Check sheet for the modelled part. Datum: model origin and axes. Units: mm. A direction names the side the tool comes from. Round coordinates to 2 decimals unless told otherwise and drop trailing zeros. Write each loop counter-clockwise with the first axis right and the second up, starting at its lowest first coordinate (ties: lowest second). Pieces come first, ordered by that corner, then holes.
Item 1: Material ranges on line 1 (Y direction, x = -26, z = 45); line 2 (Z direction, x = -27.25, y = -33.5); line 3 (X direction, y = -36.5, z = 44.9), recorded low to high.
Item 2: Cross-section at A-A on x = -26. Enter the section's corners in (y, z).
Item 3: Tool access check on faces 5 (the flat face through (-23.36, -34.51, 46.49)), 6 (the cylindrical face through (-25.26, -37.42, 44.38)). Record the directions out of +Z, -Z, +X, -X, +Y, -Y that give a thin tool (end or side, any length) a straight path to the whole face; none if there is none.
Item 4: Cross-section at B-B on z = 44.3. Enter the section's corners in (x, y).
Item 5: Go/stop test with flat-tipped pins: pin 1 Ø1.5 at (y, z) = (-38.5, 46.5) entering from +X; pin 2 Ø1.5 at (x, z) = (-27.5, 45) entering from +Y; pin 3 Ø0.5 at (x, z) = (-26.5, 46.5) entering from -Y; pin 4 Ø3 at (x, y) = (-26, -36) entering from +Z. Record where each tip stops, or that it passes through.
Item 6: Release check for a two-part mould opening along Y. For faces 1 (the flat face through (-23.39, -37.54, 46.49)), 2 (the flat face through (-29, -34, 47)), 3 (the cylindrical face through (-26.521, -32.034, 44.873)), 4 (the flat face through (-28.61, -34.46, 46.49)) record: +Y half, -Y half, draft (parallel to the pull), parting line (faces both ways), or undercut.
from build123d import *

# Parameters (mm, degrees)
SKETCH182_R     = 4
SKETCH182_R_2   = 1.6
PAD075_DEPTH    = 3.2
SKETCH183_R     = 4
PAD076_DEPTH    = 1
CHAMFER032_SIZE = 0.2


with BuildPart() as part:
    # Sketch182 → Pad075 (new body)
    with BuildSketch(Plane.XY):
        Circle(SKETCH182_R)
        Circle(SKETCH182_R_2, mode=Mode.SUBTRACT)
    extrude(amount=PAD075_DEPTH)

    # Sketch183 (on Face4 of Pad075) → Pad076 (join)
    with BuildSketch(Plane.XY.offset(3.2)):
        Circle(SKETCH183_R)
        Polygon((3.5, 0), (1.75, 3.031089), (-1.75, 3.031089), (-3.5, 0), (-1.75, -3.031089), (1.75, -3.031089), align=None, mode=Mode.SUBTRACT)
    extrude(amount=PAD076_DEPTH)

    # Chamfer032
    chamfer032_edges = [part.edges().sort_by_distance(p)[0] for p in [
        (-1.6, 0, 3.2),
        (-1.6, 0, 0),
        (-4, 0, 0),
        (-4, 0, 4.2),
    ]]
    chamfer(chamfer032_edges, length=CHAMFER032_SIZE)


with BuildPart() as part_1:
    # Body049 placement: moved
    add(part.part.moved(Location((-26, -36, 42.8))))


solid = part_1.part
Response values:
1. line 1: y = -40 to -37.6, -34.4 to -32
1. line 2: z = 42.8 to 46
1. line 3: x = -29.97 to -27.52, -24.48 to -22.03
2. outline: (-40, 43) - (-39.8, 42.8) - (-37.8, 42.8) - (-37.6, 43) - (-37.6, 45.8) - (-37.8, 46) - (-39.03, 46) - (-39.03, 47) - (-39.8, 47) - (-40, 46.8) - close; (-34.4, 43) - (-34.2, 42.8) - (-32.2, 42.8) - (-32, 43) - (-32, 46.8) - (-32.2, 47) - (-32.97, 47) - (-32.97, 46) - (-34.2, 46) - (-34.4, 45.8) - close
3. face 5: +Z
3. face 6: +Z, -Z
4. outline: circle Ø8 at (-26, -36); hole circle Ø3.2 at (-26, -36)
5. pin 1: stops at x = -22.4
5. pin 2: stops at y = -32.07
5. pin 3: stops at y = -39.99
5. pin 4: passes through
6. face 1: undercut
6. face 2: draft
6. face 3: parting line
6. face 4: undercut
